Design review of the part built by this model. Coordinates are the model's own, in mm. A direction names the side the tool comes from. Round coordinates to 2 decimals unless told otherwise and drop trailing zeros. Loops run counter-clockwise (first coordinate to the right, second up) from the corner with the lowest first, then second, coordinate; pieces in that order, holes last. Notation, with made-up numbers: (14.25, -25) - (42.25, -25) arc R17 ccw to (42.25, -14) - close; hole circle Ø8 at (-2, -32.5). An arc over 180 degrees is marked (long way). Return JSON: item names as keys, results as strings. Group by question number.
(1) For faces 1 (the cylindrical face through (2.152, -1.972, 0.088)), 2 (the cylindrical face through (3.604, 19.493, 11.446)), 3 (the cylindrical face through (1.9, 22.5, 5.9)), list the 3-axis set-ups (+Z, -Z, +X, -X, +Y, -Y) from which the entire face can be reached by the end or side of a thin tool; tool diameter is ignored.
(2) The part is to be moulded in two halves that separate along X. For faces 4 (the flat face through (3, 19, -6)), 5 (the cylindrical face through (-2.44, 28.45, -0.54)), 6 (the flat face through (0, 0, 0)), say which applies: pulls with the +X half, pulls with the -X half, needs draft (parallel to the pull), parting line crosses it, or undercut.
(3) Clearance check with flat-ended pins moving along their axes: pin 1 (3 mm diameter, centred on y = 16.5, z = 0.5, fed in from +X); pin 2 (1.5 mm diameter, centred on x = 1, z = 3, fed in from +Y); pin 3 (2.5 mm diameter, centred on x = -7.86, z = -4.54, fed in from -Y); pin 4 (2 mm diameter, centred on x = 4, y = 6, fed in from +Z). State where each tip first meets the part, or that it passes through.
(4) We need section B-B, the plane z = -4.5. Write out the cut boundary in (x, y), and give its area (3 significant figures).
(5) We need section C-C, the plane x = -3.25. Write out the cut boundary in (y, z), and give its area (3 significant figures).
(6) We need section D-D, the plane y = 23. Write out the cut boundary in (x, z).
(7) Wall thickness on L1, parallel to Y at x = 6.5, z = 0; L2, parallel to Y at x = -3, z = -0.5; L3, parallel to Z at x = -2.25, y = 26.5: over which ranges is each line inside the solid? List them lowest first. Write a range as [from, to].
(8) We need section A-A, the plane x = 0. Write out the cut boundary in (y, z) (3 decimals).
from build123d import *

# Parameters (mm, degrees)
SKETCH1_R           = 6.15
BOSS_EXTRUDE1_DEPTH = 19
SKETCH2_R           = 12
BOSS_EXTRUDE2_DEPTH = 1
SKETCH3_R           = 6.2
BOSS_EXTRUDE3_DEPTH = 5
SKETCH4_R           = 2.5
BOSS_EXTRUDE4_DEPTH = 7
SKETCH5_R           = 2
BOSS_EXTRUDE5_DEPTH = 4
SKETCH6_R           = 1.7
CUT_EXTRUDE1_DEPTH  = 29.583211856


with BuildPart() as part:
    # Sketch1 → Boss-Extrude1 (new body)
    with BuildSketch(Plane(origin=(0, 0, 0), x_dir=(1, 0, 0), z_dir=(0, 1, 0))):
        with Locations(Location((0, 0, 0), (0, 0, 270))):
            Circle(SKETCH1_R)
    extrude(amount=BOSS_EXTRUDE1_DEPTH)

    # Sketch2 → Boss-Extrude2 (add)
    with BuildSketch(Plane(origin=(0, 19, 0), x_dir=(1, 0, 0), z_dir=(0, 1, 0))):
        with Locations(Location((0, 0, 0), (0, 0, 270))):
            Circle(SKETCH2_R)
    extrude(amount=BOSS_EXTRUDE2_DEPTH)

    # Sketch3 → Boss-Extrude3 (add)
    with BuildSketch(Plane(origin=(0, 20, 0), x_dir=(1, 0, 0), z_dir=(0, 1, 0))):
        with Locations(Location((0, 0, 0), (0, 0, 270))):
            Circle(SKETCH3_R)
    extrude(amount=BOSS_EXTRUDE3_DEPTH)

    # Sketch4 → Boss-Extrude4 (add)
    with BuildSketch(Plane(origin=(0, 25, 0), x_dir=(1, 0, 0), z_dir=(0, 1, 0))):
        with Locations(Location((0, 0, 0), (0, 0, 270))):
            Circle(SKETCH4_R)
    extrude(amount=BOSS_EXTRUDE4_DEPTH)

    # Sketch5 → Boss-Extrude5 (add)
    with BuildSketch(Plane.XZ):
        with Locations(Location((-4.15, 0, 0), (0, 0, 179.999302513))):
            Circle(SKETCH5_R)
        with Locations(Location((4.15, 0, 0), (0, 0, 359.999302513))):
            Circle(SKETCH5_R)
    extrude(amount=BOSS_EXTRUDE5_DEPTH)

    # Sketch6 → Cut-Extrude1 (cut, through all)
    with BuildSketch(Plane.XZ.offset(-19)):
        with Locations(Location((0, 9.075, 0), (0, 0, 270))):
            Circle(SKETCH6_R)
        with Locations(Location((7.859180539, -4.5375, 0), (0, 0, 270))):
            Circle(SKETCH6_R)
        with Locations(Location((-7.859180539, -4.5375, 0), (0, 0, 270))):
            Circle(SKETCH6_R)
    extrude(amount=-CUT_EXTRUDE1_DEPTH, mode=Mode.SUBTRACT)


solid = part.part
Solutions:
{
 "1": {"face 1": "-Y", "face 2": "+Y, -Y", "face 3": "+Y"},
 "2": {"face 4": "needs draft", "face 5": "parting line crosses it", "face 6": "undercut"},
 "3": {"pin 1": "x = 6.15", "pin 2": "y = 32", "pin 3": "through", "pin 4": "z = 5.37"},
 "4": {"outline": "(-11.12, 19) - (-9.56, 19) - (-9.56, 20) - (-11.12, 20) - close; (-6.16, 19) - (-4.19, 19) - (-4.19, 0) - (4.19, 0) - (4.19, 19) - (6.16, 19) - (6.16, 20) - (4.26, 20) - (4.26, 25) - (-4.26, 25) - (-4.26, 20) - (-6.16, 20) - close; (9.56, 19) - (11.12, 19) - (11.12, 20) - (9.56, 20) - close", "area": "217 mm^2"},
 "5": {"outline": "(-4, -1.79) - (0, -1.79) - (0, -5.22) - (19, -5.22) - (19, -11.55) - (20, -11.55) - (20, -5.28) - (25, -5.28) - (25, 5.28) - (20, 5.28) - (20, 11.55) - (19, 11.55) - (19, 5.22) - (0, 5.22) - (0, 1.79) - (-4, 1.79) - close", "area": "289 mm^2"},
 "6": {"outline": "circle Ø12.4 at (0, 0)"},
 "7": {"L1": "[19, 20]", "L2": "[-4, 25]", "L3": "[-1.09, 1.09]"},
 "8": {"outline": "(0, -6.15) - (19, -6.15) - (19, -12) - (20, -12) - (20, -6.2) - (25, -6.2) - (25, -2.5) - (32, -2.5) - (32, 2.5) - (25, 2.5) - (25, 6.2) - (20, 6.2) - (20, 7.375) - (19, 7.375) - (19, 6.15) - (0, 6.15) - close; (19, 10.775) - (20, 10.775) - (20, 12) - (19, 12) - close"}
}
